```python
from build123d import *

# Parameters (mm, degrees)
SKETCH_W  = 2.7051
SKETCH_H  = 2.7051
PAD_DEPTH = 9.906


with BuildPart() as part:
    # Sketch → Pad (new body)
    with BuildSketch(Plane.XY):
        Polygon((0, 3.666174), (-3.175, 1.833087), (-3.175, -1.833087), (0, -3.666174), (3.175, -1.833087), (3.175, 1.833087), align=None)
        Rectangle(SKETCH_W, SKETCH_H, mode=Mode.SUBTRACT)
    extrude(amount=PAD_DEPTH)


solid = part.part
```
Geometry: final body of the model. Coordinates: model frame, mm. A direction names the side the tool comes from. Coordinates: 2 decimals unless noted, no trailing zeros. Write each loop counter-clockwise with the first axis right and the second up, starting at its lowest first coordinate (ties: lowest second). Pieces come first, ordered by that corner, then holes. Notation, with made-up numbers: M 5.25,81 L 20.25,81 A17 cw 20.25,90 Z; hole C -8.5,26 d11. An arc over 180 degrees is marked long. Use CSV: the item, a comma, the result in double quotes. Start each with the question number.
1. Ray query, probe 1 along X at (y, z) = (0.75, 2.75) (3 decimals); probe 2 along Y at (x, z) = (1, 4); probe 3 along Y at (x, z) = (0.75, 7). Return the intervals inside material, ascending.
2. Cut plane C-C on z = 4.5. Return the cut outline in (x, y) (3 decimals).
3. First-contact query: P1, Ø0.8, axis at x = -0.5, z = 7.5, coming from the +Y side; P2, Ø1, axis at x = -2.5, z = 6.5, coming from the -Y side; P3, Ø2, axis at x = -0.5, z = 3.5, coming from the -Y side. Flat tips, straight axial feed; report the tip coordinate or a pass-through.
4. Reachability of faces 1 (the face through (1.57, -2.76, 4.88)), 2 (the face through (-1.353, 0, 5)) from +Z, -Z, +X, -X, +Y, -Y: full face, straight path, thin tool, end or side. Return the list, or none.
5. Cut plane B-B on x = -0.5. Return the cut outline in (y, z).
6. Mould query, pull axis X, two halves, no side actions, for faces 3 (the face through (0, -1.353, 5)), 4 (the face through (-3.175, 0, 5)), 5 (the face through (0, -2, 0)), 6 (the face through (1.353, 0, 5)). Classes: pulls with the +X half, pulls with the -X half, needs draft (parallel to the pull), parting line crosses it, or undercut.
7. Cut plane D-D on x = 2.5. Return the cut outline in (y, z), plus the area to 3 significant figures.
8. Cut plane A-A on y = 0. Return the cut outline in (x, z) (3 decimals), plus the area to 3 significant figures.
Entries:
1,probe 1,"-3.175 to -1.353, 1.353 to 3.175"
1,probe 2,"-3.09 to -1.35, 1.35 to 3.09"
1,probe 3,"-3.23 to -1.35, 1.35 to 3.23"
2,outline,"M -3.175,-1.833 L 0,-3.666 L 3.175,-1.833 L 3.175,1.833 L 0,3.666 L -3.175,1.833 Z; hole M -1.353,-1.353 L 1.353,-1.353 L 1.353,1.353 L -1.353,1.353 Z"
3,P1,"y = 3.61"
3,P2,"y = -2.51"
3,P3,"y = -3.67"
4,face 1,"+Z, -Z, +X, -Y"
4,face 2,"+Z, -Z"
5,outline,"M -3.38,0 L -1.35,0 L -1.35,9.91 L -3.38,9.91 Z; M 1.35,0 L 3.38,0 L 3.38,9.91 L 1.35,9.91 Z"
6,face 3,"undercut"
6,face 4,"pulls with the -X half"
6,face 5,"needs draft"
6,face 6,"undercut"
7,outline,"M -2.22,0 L 2.22,0 L 2.22,9.91 L -2.22,9.91 Z"
7,area,"44.0 mm²"
8,outline,"M -3.175,0 L -1.353,0 L -1.353,9.906 L -3.175,9.906 Z; M 1.353,0 L 3.175,0 L 3.175,9.906 L 1.353,9.906 Z"
8,area,"36.1 mm²"
